from build123d import *

# Parameters (mm, degrees)
F0_R     = 12.25
F0_R_2   = 9.8
F1_DEPTH = 1.45
F2_SIZE  = 0.5
F3_R     = 0.5


with BuildPart() as f1:
    # F0 (on Front) → F1 (new body)
    with BuildSketch(Plane.XZ):
        Circle(F0_R)
        Circle(F0_R_2, mode=Mode.SUBTRACT)
    extrude(amount=F1_DEPTH)

    # F2
    f2_edges = [f1.edges().sort_by_distance(p)[0] for p in [
        (-12.25, 0, 0),
    ]]
    chamfer(f2_edges, length=F2_SIZE)

    # F3
    f3_edges = [f1.edges().sort_by_distance(p)[0] for p in [
        (-9.8, -1.45, 0),
    ]]
    fillet(f3_edges, radius=F3_R)


solid = f1.part
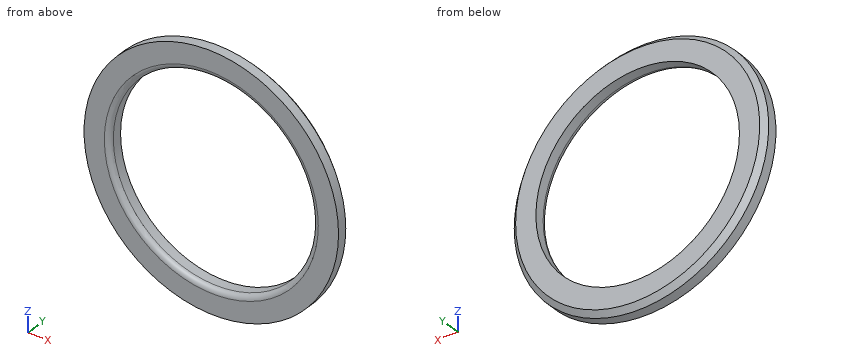
CAD build for the part. Positions are in the model's coordinates, mm. Round coordinates to 2 decimals unless told otherwise and drop trailing zeros. Write each loop counter-clockwise with the first axis right and the second up, starting at its lowest first coordinate (ties: lowest second). Pieces come first, ordered by that corner, then holes.
(1) Drop a flat-ended pin along its axis: P1, Ø12, axis at x = 0, z = 0, coming from the -Y side. Give the stop position or say it passes through.
(2) Slice it at A-A, the plane x = 0. Write the cut outline in (y, z), and give its area (3 significant figures).
(3) Probe line 1 along Z through (x, y) = (0, -0.6); line 2 along Z through (x, y) = (4.5, -0.75); line 3 along X through (y, z) = (-0.6, 5.5). List the from-to ranges inside material, lowest first.
(4) Slice it at B-B, the plane z = 0. Write the cut outline in (x, y), and give its area (3 significant figures).
From the geometry:
1. P1: passes through
2. outline: (-1.45, -12.25) - (-0.5, -12.25) - (0, -11.75) - (0, -9.8) - (-0.95, -9.8) arc R0.5 ccw to (-1.45, -10.3) - close; (-1.45, 10.3) arc R0.5 ccw to (-0.95, 9.8) - (0, 9.8) - (0, 11.75) - (-0.5, 12.25) - (-1.45, 12.25) - close
2. area: 6.75 mm2
3. line 1: z = -12.25 to -9.8, 9.8 to 12.25
3. line 2: z = -11.39 to -8.71, 8.71 to 11.39
3. line 3: x = -10.95 to -8.11, 8.11 to 10.95
4. outline: (-12.25, -1.45) - (-10.3, -1.45) arc R0.5 ccw to (-9.8, -0.95) - (-9.8, 0) - (-11.75, 0) - (-12.25, -0.5) - close; (9.8, -0.95) arc R0.5 ccw to (10.3, -1.45) - (12.25, -1.45) - (12.25, -0.5) - (11.75, 0) - (9.8, 0) - close
4. area: 6.75 mm2
